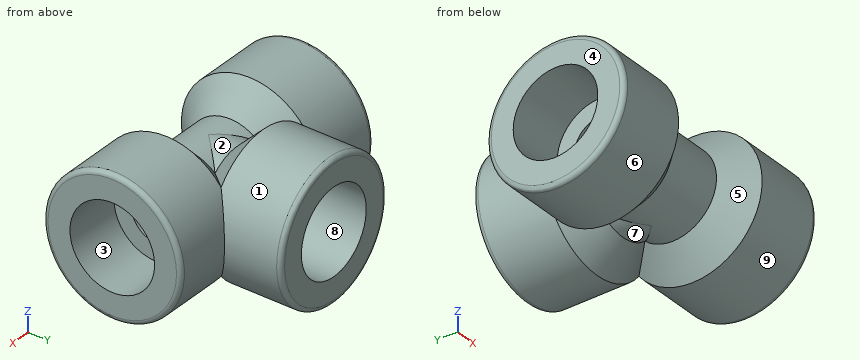
from build123d import *

# Parameters (mm, degrees)
CIRPATTERN2_COUNT       = 3
CIRPATTERN2_ANGLE       = 180
SKETCH4_R               = 4.191
CUT_EXTRUDE1_DEPTH      = 32.976017529
CUT_EXTRUDE1_DEPTH_BACK = 32.976017529
SKETCH5_R               = 4.191
CUT_EXTRUDE2_DEPTH      = 32.976017529


with BuildPart() as part:
    # Sketch2 → Revolve1 (revolve)
    with BuildSketch(Plane.XY, mode=Mode.PRIVATE) as revolve1_sk:
        with BuildLine():
            Line((-21.082, -7.112), (-11.43, -7.112))
            Line((-11.43, -7.112), (-11.43, -4.191))
            Line((-11.43, -4.191), (0, -4.191))
            Line((0, -4.191), (0, -7.2136))
            Line((0, -7.2136), (-4.81965, -7.2136))
            Line((-4.81965, -7.2136), (-9.16305, -11.557))
            Line((-9.16305, -11.557), (-20.32635, -11.557))
            ThreePointArc((-20.32635, -11.557), (-20.860675239, -11.335675239), (-21.082, -10.80135))
            Line((-21.082, -10.80135), (-21.082, -7.112))
        make_face()
    revolve(revolve1_sk.sketch.rotate(Axis((0, 0, 0), (-1, 0, 0)), 180), axis=Axis((0, 0, 0), (-1, 0, 0)))


with BuildPart() as cirpattern2_1:
    # CirPattern2: pattern copy
    add(part.part.rotate(Axis((0, 0, 0), (0, 0, -1)), 1 * CIRPATTERN2_ANGLE / (CIRPATTERN2_COUNT - 1)))

    # Sketch4 → Cut-Extrude1 (cut, two sides)
    with BuildSketch(Plane(origin=(0, 0, 0), x_dir=(0, 0, -1), z_dir=(1, 0, 0))) as cut_extrude1_sk:
        with Locations(Location((0, 0, 0), (0, 0, 270))):
            Circle(SKETCH4_R)
    extrude(amount=CUT_EXTRUDE1_DEPTH, mode=Mode.SUBTRACT)
    extrude(cut_extrude1_sk.sketch, amount=-CUT_EXTRUDE1_DEPTH_BACK, mode=Mode.SUBTRACT)


with BuildPart() as cirpattern2_2:
    # CirPattern2: pattern copy
    add(part.part.rotate(Axis((0, 0, 0), (0, 0, -1)), 2 * CIRPATTERN2_ANGLE / (CIRPATTERN2_COUNT - 1)))


with BuildPart() as part_1:
    add(part.part)

    # Combine1: union CirPattern2_1, CirPattern2_2
    add(cirpattern2_1.part)
    add(cirpattern2_2.part)

    # Sketch5 → Cut-Extrude2 (cut, through all)
    with BuildSketch(Plane(origin=(0, 0, 0), x_dir=(1, 0, 0), z_dir=(0, 1, 0))):
        Circle(SKETCH5_R)
    extrude(amount=CUT_EXTRUDE2_DEPTH, mode=Mode.SUBTRACT)


solid = part_1.part
Geometry: final body of the model. Coordinates: model frame, mm. Face numbers are marked on the shaded views. A direction names the side the tool comes from. Round coordinates to 2 decimals unless told otherwise and drop trailing zeros. Loops run counter-clockwise (first coordinate to the right, second up) from the corner with the lowest first, then second, coordinate; pieces in that order, holes last. Notation, with made-up numbers: (61.25, -2) -> (114.25, -2) arc R15 ccw to (114.25, 15) -> close; hole circle Ø2 at (-24.75, -15). An arc over 180 degrees is marked (long way). One line per question, with ' | ' between items. Start each with the question number.
1. Section B-B on z = 0. Count the separate pieces of the cut face and the enclosed holes in it, and give its area (3 significant figures).
2. Section A-A on x = 0. Output: boundary loops of the cut face in (y, z), and give its area (3 significant figures).
3. Section C-C on y = 14. Output: boundary loops of the cut face in (x, z).
4. Set-up query: the marked faces 5, 6, 7, 8 and 9. Return all of +Z, -Z, +X, -X, +Y, -Y with unobstructed straight access to the full face (end or side cutting, diameter ignored); none if empty.
5. Line query: line 1 along Z through (x, y) = (-15, 0); line 2 along Z through (x, y) = (-4, 0); line 3 along Y through (x, z) = (-12.5, -3.25). Output: solid intervals per line, ascending. Write a range as [from, to].
6. Mould query, pull axis X, two halves, no side actions, for the marked faces 1, 2, 3 and 4. Classes: pulls with the +X half, pulls with the -X half, needs draft (parallel to the pull), parting line crosses it, or undercut.
7. Contact query for flat-ended pins moving along their axis: pin 1 (7.5 mm diameter, centred on x = 0, z = 0, fed in from -Y); pin 2 (4.5 mm diameter, centred on x = 0.5, z = -3.5, fed in from +Y); pin 3 (12 mm diameter, centred on x = 13.5, y = 11.5, fed in from -Z); pin 4 (6.5 mm diameter, centred on y = 0, z = 0, fed in from +X). Output: stop coordinate, or through.
Returned:
1) separate pieces: 3 | enclosed holes: 0 | area: 469 mm2
2) outline: (0, -7.21) -> (4.82, -7.21) -> (9.16, -11.56) -> (20.33, -11.56) arc R0.76 ccw to (21.08, -10.8) -> (21.08, -7.11) -> (11.43, -7.11) -> (11.43, -4.19) -> (0, -4.19) arc R4.19 cw to (0, 4.19) -> (11.43, 4.19) -> (11.43, 7.11) -> (21.08, 7.11) -> (21.08, 10.8) arc R0.76 ccw to (20.33, 11.56) -> (9.16, 11.56) -> (4.82, 7.21) -> (0, 7.21) arc R7.21 ccw to start | area: 247 mm2
3) outline: circle Ø23.11 at (0, 0); hole circle Ø14.22 at (0, 0)
4) face 5: none | face 6: -X | face 7: -Z | face 8: +Y | face 9: +X
5) line 1: z = [-11.56, -7.11], [7.11, 11.56] | line 2: z = [-7.21, -4.19], [4.19, 7.21] | line 3: y = [-11.09, -6.33], [6.33, 11.09]
6) face 1: parting line crosses it | face 2: undercut | face 3: needs draft | face 4: pulls with the -X half
7) pin 1: stops at y = -7.21 | pin 2: stops at y = 11.43 | pin 3: stops at z = -10.16 | pin 4: passes through
